```python
from build123d import *

# Parameters (mm, degrees)
SKETCH1_R           = 1.75
BOSS_EXTRUDE1_DEPTH = 7
SKETCH2_W           = 3
SKETCH2_H           = 3
CUT_EXTRUDE1_DEPTH  = 17.170961629


with BuildPart() as part:
    # Sketch1 → Boss-Extrude1 (new body)
    with BuildSketch(Plane.XY):
        with BuildLine():
            Line((-6.873863542, 3), (-3.818813079, 10))
            ThreePointArc((-3.818813079, 10), (0, 12.5), (3.818813079, 10))
            Line((3.818813079, 10), (6.873863542, 3))
            ThreePointArc((6.873863542, 3), (0, -7.5), (-6.873863542, 3))
        make_face()
        Circle(SKETCH1_R, mode=Mode.SUBTRACT)
    extrude(amount=BOSS_EXTRUDE1_DEPTH)

    # Sketch2 → Cut-Extrude1 (cut, through all)
    with BuildSketch(Plane.XY.offset(7)):
        with Locations((0, 4.5)):
            Rectangle(SKETCH2_W, SKETCH2_H)
        with Locations((4.5, 0)):
            Rectangle(SKETCH2_W, SKETCH2_H)
    extrude(amount=-CUT_EXTRUDE1_DEPTH, mode=Mode.SUBTRACT)


solid = part.part
```
The model under review builds one solid part; all positions refer to its coordinate system, in mm. A direction names the side the tool comes from. Give positions to 0.01 mm unless a question says otherwise; leave off trailing zeros. Write each loop counter-clockwise with the first axis right and the second up, starting at its lowest first coordinate (ties: lowest second). Pieces come first, ordered by that corner, then holes. Notation, with made-up numbers: M 13.25,65 L 29.25,65 A23 cw 29.25,104 Z; hole C 12.25,44 d4. An arc over 180 degrees is marked long. Answer in a Markdown table with one row per item.
Item 1: Add section C-C on z = 4. Give the boundary of the cut face in (x, y).
Check sheet entries:
| item | result |
|---|---|
| outline | M -6.87,3 A7.5 ccw long 6.87,3 L 3.82,10 A4.17 ccw -3.82,10 Z; hole C 0,0 d3.5; hole M -1.5,3 L 1.5,3 L 1.5,6 L -1.5,6 Z; hole M 3,-1.5 L 6,-1.5 L 6,1.5 L 3,1.5 Z |
Item 2: Tool access review of faces 5 (the face through (4, 1.5, 4)), 6 (the face through (5.325, 6.549, 3.451)): name each direction out of +Z, -Z, +X, -X, +Y, -Y from which nothing blocks a thin tool from reaching the whole face with its end or side.
Check sheet entries:
| item | result |
|---|---|
| face 5 | +Z, -Z |
| face 6 | +Z, -Z, +X, +Y |
Item 3: For P1, Ø2.5, axis at y = 4.5, z = 4.5, coming from the -X side; P2, Ø0.9, axis at y = 5, z = 3, coming from the +X side; P3, Ø3, axis at x = 0, y = 0, coming from the -Z side; P4, Ø2.5, axis at x = 5, z = 5, coming from the -Y side, all flat-tipped, find the tip position at first contact; note any pin that passes through.
Check sheet entries:
| item | result |
|---|---|
| P1 | x = -6.76 |
| P2 | x = 6.2 |
| P3 | through |
| P4 | y = -6.5 |
Item 4: Draft analysis for pull direction Y (two halves, no side actions). For faces 1 (the face through (-5.37, 6.45, 3.45)), 2 (the face through (0.208, -7.497, 3.451)), 3 (the face through (0.1, 2.6, 0)), 4 (the face through (3, 0, 4)), state which applies: +Y half, -Y half, draft (parallel to the pull), parting line (faces both ways), or undercut.
Check sheet entries:
| item | result |
|---|---|
| face 1 | +Y half |
| face 2 | parting line |
| face 3 | draft |
| face 4 | undercut |
Item 5: Add section B-B on y = 0. Give the boundary of the cut face in (x, z).
Check sheet entries:
| item | result |
|---|---|
| outline | M -7.5,0 L -1.75,0 L -1.75,7 L -7.5,7 Z; M 1.75,0 L 3,0 L 3,7 L 1.75,7 Z; M 6,0 L 7.5,0 L 7.5,7 L 6,7 Z |
Item 6: Add section D-D on x = 3.5. Give the boundary of the cut face in (y, z), plus the area to 3 significant figures.
Check sheet entries:
| item | result |
|---|---|
| outline | M -6.63,0 L -1.5,0 L -1.5,7 L -6.63,7 Z; M 1.5,0 L 10.59,0 L 10.59,7 L 1.5,7 Z |
| area | 99.6 mm2 |
Item 7: Add section A-A on x = 0. Give the boundary of the cut face in (y, z), plus the area to 3 significant figures.
Check sheet entries:
| item | result |
|---|---|
| outline | M -7.5,0 L -1.75,0 L -1.75,7 L -7.5,7 Z; M 1.75,0 L 3,0 L 3,7 L 1.75,7 Z; M 6,0 L 12.5,0 L 12.5,7 L 6,7 Z |
| area | 94.5 mm2 |
Item 8: For line 1 along Y through (x, z) = (0, 2.75); line 2 along Y through (x, z) = (-0.75, 5.75); line 3 along X through (y, z) = (3.75, 1), list the stretches that pass through material, from the lowest coordinate up.
Check sheet entries:
| item | result |
|---|---|
| line 1 | -7.5 to -1.75, 1.75 to 3, 6 to 12.5 |
| line 2 | -7.46 to -1.58, 1.58 to 3, 6 to 12.43 |
| line 3 | -6.55 to -1.5, 1.5 to 6.55 |
